Check sheet for the modelled part. Datum: model origin and axes. Units: mm. Face numbers are marked on the shaded views. A direction names the side the tool comes from. Coordinates: 2 decimals unless noted, no trailing zeros. Order: outer loops, then holes, each group sorted by start corner. A loop starts at its lowest first (then second) coordinate and runs counter-clockwise, first axis right, second up.
1. Thickness scan on line 1 (Y direction, x = -13.65, z = 12.5); line 2 (Y direction, x = -13.5, z = 12.5); line 3 (Y direction, x = 89.5, z = 20.5). Record the ranges inside material, lowest first.
2. Set-up check for the marked faces 4, 5 and 6: record each of +Z, -Z, +X, -X, +Y, -Y from which the full face is reachable in a straight line by a thin tool's end or side.
3. Gauge pin test, flat ends, axial feed: pin 1 Ø12 at (x, y) = (31, 26.5) entering from -Z; pin 2 Ø4 at (x, z) = (7, 2.5) entering from -Y; pin 3 Ø2.5 at (y, z) = (24, 2) entering from +X. Record the tip position at first contact, or that the pin passes through.
4. Cross-section at A-A (y = 8.5). Enter the section's corners in (x, z).
5. Cross-section at B-B (z = 12). Count the separate pieces of the cut face and the enclosed holes in it, then the cut area to 3 significant figures.
6. Draft check along Y on the marked faces 1, 2 and 3. Enter one of: released by +Y, released by -Y, zero draft, split by the parting line, or undercut.
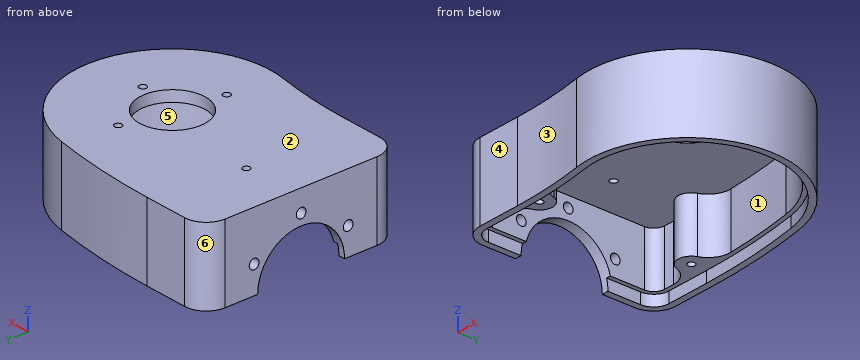
```python
from build123d import *

# Parameters (mm, degrees)
EXTRUDE_1_DEPTH        = 35
CUT_EXTRUDE_1_DEPTH    = 30
SKETCH_3_R             = 20
SKETCH_3_R_2           = 2.25
CUT_EXTRUDE_2_DEPTH    = 5
CUT_EXTRUDE_3_REACH    = 37
SKETCH_4_R             = 15
CUT_EXTRUDE_5_DEPTH    = 5
SKETCH_8_R             = 6
EXTRUDE_2_DEPTH        = 25
FILLET_1_R             = 10
HOLE_WIZARD_M4_2_D     = 3.3
HOLE_WIZARD_M4_2_DEPTH = 11.5
HOLE_WIZARD_M4_2_TIP   = 0.991420021
HOLE_WIZARD_M4_3_D     = 3.3
HOLE_WIZARD_M4_3_DEPTH = 11.5
HOLE_WIZARD_M4_3_TIP   = 0.991420021


with BuildPart() as part:
    # 스케치1 → 보스-돌출1 (new body)
    with BuildSketch(Plane.XY):
        with BuildLine():
            Line((-5, 45), (15, 45))
            ThreePointArc((15, 45), (40.275165397, 43.896462447), (65.357971523, 40.594248374))
            ThreePointArc((65.357971523, 40.594248374), (101.860152414, -11.536268507), (49.729635533, -48.038449398))
            ThreePointArc((49.729635533, -48.038449398), (32.43114855, -45.761060382), (15, -45))
            Line((15, -45), (-5, -45))
            ThreePointArc((-5, -45), (-12.071067812, -42.071067812), (-15, -35))
            Line((-15, -35), (-15, 35))
            ThreePointArc((-15, 35), (-12.071067812, 42.071067812), (-5, 45))
        make_face()
    extrude(amount=EXTRUDE_1_DEPTH)

    # 스케치2 → 컷-돌출1 (cut)
    with BuildSketch(Plane(origin=(0, 0, 0), x_dir=(-1, 0, 0), z_dir=(0, 0, -1))):
        with BuildLine():
            Line((-15, -40), (5, -40))
            ThreePointArc((5, -40), (8.535533906, -38.535533906), (10, -35))
            Line((10, -35), (10, 35))
            ThreePointArc((10, 35), (8.535533906, 38.535533906), (5, 40))
            Line((5, 40), (-15, 40))
            ThreePointArc((-15, 40), (-39.839386683, 38.915488956), (-64.489730635, 35.670209608))
            ThreePointArc((-64.489730635, 35.670209608), (-96.936113649, -10.668027619), (-50.597876422, -43.114410632))
            ThreePointArc((-50.597876422, -43.114410632), (-32.866927263, -40.780086891), (-15, -40))
        make_face()
    extrude(amount=-CUT_EXTRUDE_1_DEPTH, mode=Mode.SUBTRACT)

    # 스케치3 → 컷-돌출2 (cut)
    with BuildSketch(Plane.ZY.offset(15)):
        Circle(SKETCH_3_R)
        with Locations((12.5, 21.650635095)):
            Circle(SKETCH_3_R_2)
        with Locations((25, 0)):
            Circle(SKETCH_3_R_2)
        with Locations((12.5, -21.650635095)):
            Circle(SKETCH_3_R_2)
    extrude(amount=-CUT_EXTRUDE_2_DEPTH, mode=Mode.SUBTRACT)

    # 스케치4 → 컷-돌출3 (cut, up to next)
    with BuildSketch(Plane.XY.offset(35), mode=Mode.PRIVATE) as cut_extrude_3_sk1:
        with Locations((57.543803528, -3.722100512)):
            Circle(SKETCH_4_R)
    cut_extrude_3_tool1 = extrude(cut_extrude_3_sk1.sketch, amount=-CUT_EXTRUDE_3_REACH, mode=Mode.PRIVATE) & part.part
    add(cut_extrude_3_tool1.solids().sort_by_distance((57.543804, -3.722101, 35))[0], mode=Mode.SUBTRACT)

    # 스케치6 → 컷-돌출5 (cut)
    with BuildSketch(Plane(origin=(0, 0, 0), x_dir=(-1, 0, 0), z_dir=(0, 0, -1))):
        with BuildLine():
            Line((10, 21.02711573), (10, 19.021261947))
            Line((10, 19.021261947), (12, 19.021261947))
            Line((12, 19.021261947), (12, 21.02711573))
            Line((12, 21.02711573), (12, 35))
            ThreePointArc((12, 35), (9.949747468, 39.949747468), (5, 42))
            Line((5, 42), (-15, 42))
            ThreePointArc((-15, 42), (-40.013698169, 40.907878352), (-64.83702699, 37.639825115))
            ThreePointArc((-64.83702699, 37.639825115), (-98.905729155, -11.015323974), (-50.250580066, -45.084026139))
            ThreePointArc((-50.250580066, -45.084026139), (-32.692615778, -42.772476287), (-15, -42))
            Line((-15, -42), (5, -42))
            ThreePointArc((5, -42), (9.949747468, -39.949747468), (12, -35))
            Line((12, -35), (12, -19.081512787))
            Line((12, -19.081512787), (10, -19.081512787))
            Line((10, -19.081512787), (10, -35))
            ThreePointArc((10, -35), (8.535533906, -38.535533906), (5, -40))
            Line((5, -40), (-15, -40))
            ThreePointArc((-15, -40), (-32.866927263, -40.780086891), (-50.597876422, -43.114410632))
            ThreePointArc((-50.597876422, -43.114410632), (-96.936113649, -10.668027619), (-64.489730635, 35.670209608))
            ThreePointArc((-64.489730635, 35.670209608), (-39.839386683, 38.915488956), (-15, 40))
            Line((-15, 40), (5, 40))
            ThreePointArc((5, 40), (8.535533906, 38.535533906), (10, 35))
            Line((10, 35), (10, 21.02711573))
        make_face()
    extrude(amount=-CUT_EXTRUDE_5_DEPTH, mode=Mode.SUBTRACT)

    # 스케치8 → 보스-돌출2 (add)
    with BuildSketch(Plane(origin=(0, 0, 30), x_dir=(-1, 0, 0), z_dir=(0, 0, -1))):
        with Locations((-15, 35)):
            Circle(SKETCH_8_R)
        with Locations((-15, -35)):
            Circle(SKETCH_8_R)
    extrude(amount=EXTRUDE_2_DEPTH)

    # 필렛1
    fillet_1_edges = [part.edges().sort_by_distance(p)[0] for p in [
        (18.346048824, 39.980357143, 17.5),
        (11.68337521, 40, 17.5),
        (18.276798635, -40.026190476, 17.5),
        (11.68337521, -40, 17.5),
    ]]
    fillet(fillet_1_edges, radius=FILLET_1_R)

    # M4 나사 구멍2
    with Locations(Plane(origin=(0, 0, 30), x_dir=(-1, 0, 0), z_dir=(0, 0, -1))):
        with Locations((-61.364063437, 17.943670054), (-77.239958589, -7.195064065), (-53.72354362, -25.387871078), (-8.303415878, 4.960308371)):
            Hole(HOLE_WIZARD_M4_2_D / 2, depth=HOLE_WIZARD_M4_2_DEPTH)
            with Locations((0, 0, -(HOLE_WIZARD_M4_2_DEPTH + HOLE_WIZARD_M4_2_TIP / 2))):  # 118° drill point
                Cone(0, HOLE_WIZARD_M4_2_D / 2, HOLE_WIZARD_M4_2_TIP, mode=Mode.SUBTRACT)

    # M4 나사 구멍3
    with Locations(Plane(origin=(0, 0, 5), x_dir=(-1, 0, 0), z_dir=(0, 0, -1))):
        with Locations((-15, 35), (-15, -35)):
            Hole(HOLE_WIZARD_M4_3_D / 2, depth=HOLE_WIZARD_M4_3_DEPTH)
            with Locations((0, 0, -(HOLE_WIZARD_M4_3_DEPTH + HOLE_WIZARD_M4_3_TIP / 2))):  # 118° drill point
                Cone(0, HOLE_WIZARD_M4_3_D / 2, HOLE_WIZARD_M4_3_TIP, mode=Mode.SUBTRACT)


solid = part.part
```
Data:
1. line 1: y = -40.02 to -23.9, -19.4 to -15.61, 15.61 to 19.4, 23.9 to 40.02
1. line 2: y = -40.27 to -23.9, -19.4 to -15.61, 15.61 to 19.4, 23.9 to 40.27
1. line 3: y = -35.4 to -27.78, 20.34 to 27.96
2. face 4: +Z, -Z, -X, -Y
2. face 5: -Z
2. face 6: +Z, -Z, -X, +Y
3. pin 1: stops at z = 30
3. pin 2: stops at y = -45
3. pin 3: stops at x = 93.93
4. outline: (-15, 18.1) - (-10, 18.1) - (-10, 30) - (48.85, 30) - (48.85, 35) - (-15, 35) - close; (66.24, 30) - (95.63, 30) - (95.63, 5) - (97.73, 5) - (97.73, 0) - (100.85, 0) - (100.85, 35) - (66.24, 35) - close
5. separate pieces: 3
5. enclosed holes: 2
5. area: 1,840 mm2
6. face 1: undercut
6. face 2: zero draft
6. face 3: released by -Y
